Here's the drawing with two shaded views (mm, measured from the low corner). I have some questions. Round coordinates to 2 decimals unless told otherwise and drop trailing zeros. Write each loop counter-clockwise with the first axis right and the second up, starting at its lowest first coordinate (ties: lowest second). Pieces come first, ordered by that corner, then holes. Notation, with made-up numbers: (-16.5, 9.25) -> (-6.5, 9.25) arc R19 ccw to (-6.5, 30.25) -> close; hole circle Ø2 at (70.25, 76). An arc over 180 degrees is marked (long way). Use CSV: the item, a comma, the result in double quotes.
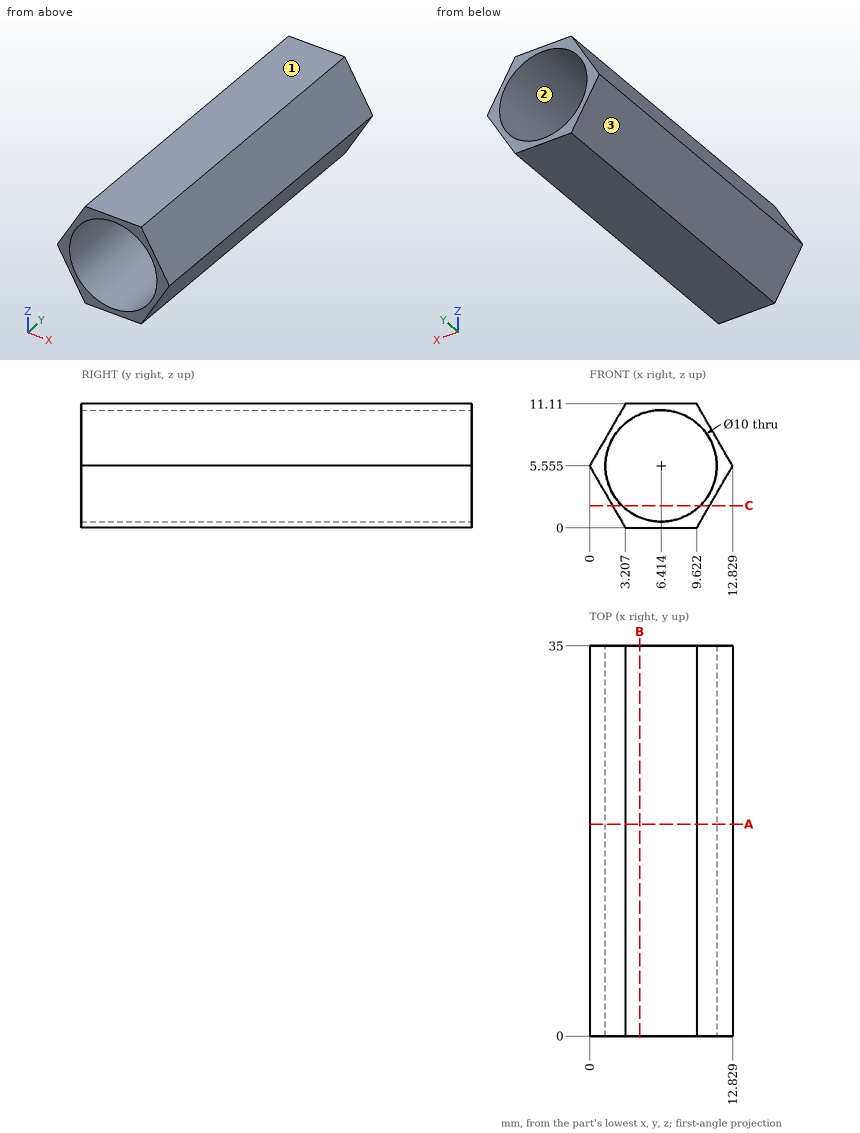
Q1. Will these pins go through, and if not, where does the flat tip stop? P1, Ø5, axis at y = 17.5, z = 2.5, coming from the +X side; P2, Ø5, axis at x = 4.5, z = 6.5, coming from the +Y side; P3, Ø6, axis at y = 17.5, z = 4, coming from the -X side.
Resolved:
P1,"stops at x = 12.51"
P2,"passes through"
P3,"stops at x = 0"
Q2. Suppose I cut it at B-B (x = 4.5). Write out the boundary of the cut face in (y, z).
Resolved:
outline,"(0, 0) -> (35, 0) -> (35, 0.94) -> (0, 0.94) -> close; (0, 10.17) -> (35, 10.17) -> (35, 11.11) -> (0, 11.11) -> close"
Q3. Suppose I cut it at A-A (y = 19). Write out the boundary of the cut face in (x, z) (1 decimal).
Resolved:
outline,"(0, 5.6) -> (3.2, 0) -> (9.6, 0) -> (12.8, 5.6) -> (9.6, 11.1) -> (3.2, 11.1) -> close; hole circle Ø10 at (6.4, 5.6)"
Q4. Please list where these lines run through material, in increasing order: probe 1 along X at (y, z) = (30, 6.5) (1 decimal); probe 2 along X at (y, z) = (19, 8.75) (1 decimal); probe 3 along Z at (x, y) = (7.5, 18.5) (1 decimal).
Resolved:
probe 1,"x = 0.5 to 1.5, 11.3 to 12.3"
probe 2,"x = 1.8 to 2.6, 10.3 to 11"
probe 3,"z = 0 to 0.7, 10.4 to 11.1"
Q5. Suppose I cut it at C-C (z = 2). Write out the boundary of the cut face in (x, y).
Resolved:
outline,"(2.05, 0) -> (2.9, 0) -> (2.9, 35) -> (2.05, 35) -> close; (9.93, 0) -> (10.78, 0) -> (10.78, 35) -> (9.93, 35) -> close"
Q6. If we mould it in two halves opening along Z, with no side actions, what happens to the marked faces 1, 2 and 3? For each: released by +Z, released by -Z, zero draft, split by the parting line, or undercut.
Resolved:
face 1,"released by +Z"
face 2,"undercut"
face 3,"released by -Z"
